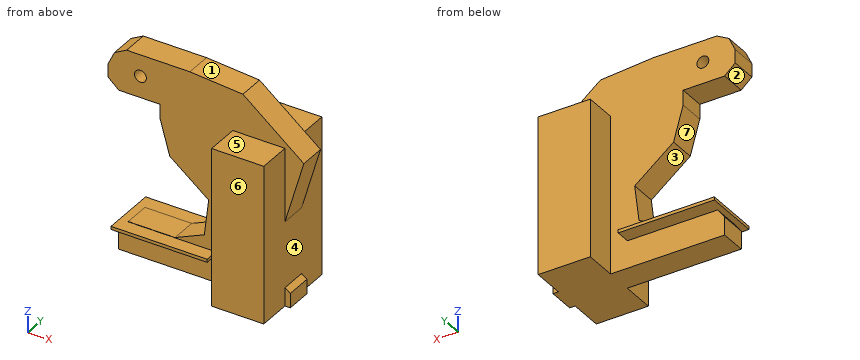
```python
from build123d import *

# Parameters (mm, degrees)
F0_R     = 2.843531
F1_DEPTH = 12.6
F3_W     = 43.916751
F3_H     = 75.827486
F4_DEPTH = 25
F6_W     = 46.128386
F6_H     = 26.223674
F7_DEPTH = 1.5


with BuildPart() as f1:
    # F0 (on Front) → F1 (new body)
    with BuildSketch(Plane.XZ):
        Polygon((52.60532, -59.951108), (45.654465, -55.053912), (49.761787, -27.250502), (59.082251, 4.660231), (29.857071, 28.040372), (4.423271, 30.094033), (-25.907725, 30.094033), (-31.752758, 26.934555), (-34.754265, 20.615598), (-34.754265, 14.138667), (-29.699098, 9.557423), (-9.794383, 9.557423), (-9.794383, 2.448596), (-5.21314, -13.822719), (13.427783, -28.514294), (11.374122, -45.891427), (-2.685557, -52.052412), (-25.117856, -52.052412), (-29.699098, -58.21339), (-29.699098, -66.901959), (52.60532, -66.901959), align=None)
        with Locations((-19.272819, 19.825729)):
            Circle(F0_R, mode=Mode.SUBTRACT)
    extrude(amount=F1_DEPTH)

    # F3 (on offset) → F4 (join)
    with BuildSketch(Plane.YZ.offset(25)):
        with Locations((-6.634905, -28.988216)):
            Rectangle(F3_W, F3_H)
    extrude(amount=F4_DEPTH)

    # F6 (on offset) → F7 (join)
    with BuildSketch(Plane.XY.offset(-52.2)):
        with Locations((-6.160983, -6.081997)):
            Rectangle(F6_W, F6_H)
    extrude(amount=-F7_DEPTH)


solid = f1.part
```
For this review, take the finished solid that the model builds, in its own axes (mm). Face numbers are marked on the shaded views. A direction names the side the tool comes from. Round coordinates to 2 decimals unless told otherwise and drop trailing zeros. Write each loop counter-clockwise with the first axis right and the second up, starting at its lowest first coordinate (ties: lowest second). Pieces come first, ordered by that corner, then holes. Notation, with made-up numbers: (68.25, 27) - (96.25, 27) arc R23 ccw to (96.25, 66) - close; hole circle Ø11 at (-32.5, 48.25). An arc over 180 degrees is marked (long way). Write each question's results on one line, items separated by ' | '.
Item 1: Draft analysis for pull direction Z (two halves, no side actions). For the marked faces 1, 2 and 3, state which applies: pulls with the +Z half, pulls with the -Z half, needs draft (parallel to the pull), parting line crosses it, or undercut.
Calculated:
face 1: pulls with the +Z half | face 2: pulls with the -Z half | face 3: undercut
Item 2: Take a section at B-B on x = -27.5. State the section outline as (y, z) points, then the cut area to 3 significant figures.
Calculated:
outline: (-19.19, -53.7) - (7.03, -53.7) - (7.03, -52.2) - (-19.19, -52.2) - close; (-12.6, -66.9) - (0, -66.9) - (0, -55.26) - (-12.6, -55.26) - close; (-12.6, 9.56) - (0, 9.56) - (0, 29.23) - (-12.6, 29.23) - close | area: 434 mm^2
Item 3: For pin 1 (5.5 mm diameter, centred on y = -4, z = 4, fed in from -X); pin 2 (1 mm diameter, centred on x = -6, y = 1, fed in from +Z); pin 3 (8 mm diameter, centred on y = -9, z = -6.5, fed in from -X), all flat-tipped, find the tip position at first contact; note any pin that passes through.
Calculated:
pin 1: stops at x = -9.79 | pin 2: stops at z = -52.2 | pin 3: stops at x = -8.4
Item 4: To check wall thickness, follow line 1 along Z through (x, y) = (-19, -5); line 2 along Y through (x, z) = (-5.5, -55); line 3 along X through (y, z) = (-20.5, -6.5). State the ranges of each line that lie inside material, in increasing order. Write a range as from..to.
Calculated:
line 1: z = -66.9..-52.05, 9.56..17, 22.66..30.09 | line 2: y = -12.6..0 | line 3: x = 25..50
Item 5: Take a section at C-C on x = 6.5. State the section outline as (y, z) points.
Calculated:
outline: (-19.19, -53.7) - (-12.6, -53.7) - (-12.6, -66.9) - (0, -66.9) - (0, -53.7) - (7.03, -53.7) - (7.03, -52.2) - (0, -52.2) - (0, -48.03) - (-12.6, -48.03) - (-12.6, -52.2) - (-19.19, -52.2) - close; (-12.6, -23.05) - (0, -23.05) - (0, 29.93) - (-12.6, 29.93) - close
Item 6: For the marked faces 4, 5, 6 and 7, list the 3-axis set-ups (+Z, -Z, +X, -X, +Y, -Y) from which the entire face can be reached by the end or side of a thin tool; tool diameter is ignored.
Calculated:
face 4: +X | face 5: +Z, +X, -X, -Y | face 6: +Z, -Z, +X, -X, -Y | face 7: -X, +Y, -Y
Item 7: Take a section at A-A on y = -15.5. State the section outline as (x, z) points, then the cut area to 3 significant figures.
Calculated:
outline: (-29.23, -53.7) - (16.9, -53.7) - (16.9, -52.2) - (-29.23, -52.2) - close; (25, -66.9) - (50, -66.9) - (50, 8.93) - (25, 8.93) - close | area: 1,960 mm^2
Item 8: Take a section at D-D on y = -7.5. State the section outline as (x, z) points.
Calculated:
outline: (-34.75, 14.14) - (-29.7, 9.56) - (-9.79, 9.56) - (-9.79, 2.45) - (-5.21, -13.82) - (13.43, -28.51) - (11.37, -45.89) - (-2.69, -52.05) - (-25.12, -52.05) - (-25.23, -52.2) - (-29.23, -52.2) - (-29.23, -53.7) - (-26.34, -53.7) - (-29.7, -58.21) - (-29.7, -66.9) - (52.61, -66.9) - (52.61, -59.95) - (50, -58.12) - (50, -26.43) - (59.08, 4.66) - (29.86, 28.04) - (4.42, 30.09) - (-25.91, 30.09) - (-31.75, 26.93) - (-34.75, 20.62) - close; hole circle Ø5.69 at (-19.27, 19.83)
